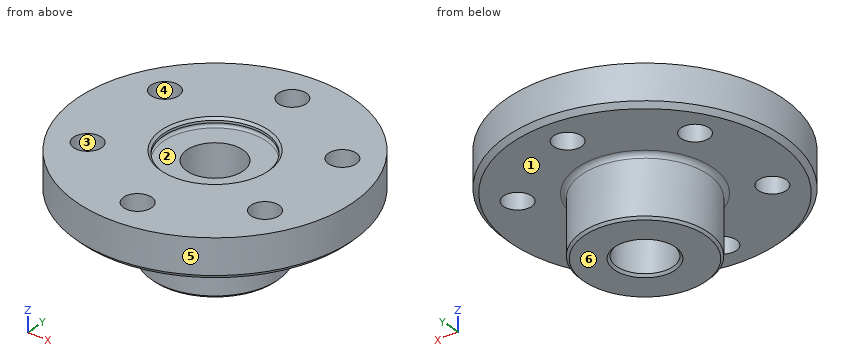
from build123d import *

# Parameters (mm, degrees)
CUT_EXTRUDE1_REACH = 89.396
SKETCH2_R          = 6
CIRPATTERN1_COUNT  = 6
FILLET1_R          = 2
CHAMFER1_SIZE      = 1
CHAMFER2_SIZE      = 2


with BuildPart() as part:
    # Sketch1 → Revolve1 (revolve)
    with BuildSketch(Plane(origin=(0, 0, 0), x_dir=(0, 0, -1), z_dir=(1, 0, 0)), mode=Mode.PRIVATE) as revolve1_sk:
        with BuildLine():
            Line((1.376389422, 12), (1.376389422, 22))
            ThreePointArc((1.376389422, 22), (0.376389422, 23), (-0.623610578, 22))
            Line((-0.623610578, 22), (-2.623610578, 22))
            Line((-2.623610578, 22), (-2.623610578, 59))
            Line((-2.623610578, 59), (14.376389422, 59))
            Line((14.376389422, 59), (14.376389422, 27))
            Line((14.376389422, 27), (40.376389422, 27))
            Line((40.376389422, 27), (40.376389422, 12))
            Line((40.376389422, 12), (1.376389422, 12))
        make_face()
    revolve(revolve1_sk.sketch.rotate(Axis((0, 0, 9.001223373), (0, 0, -1)), 90), axis=Axis((0, 0, 9.001223373), (0, 0, -1)))

    # Sketch2 → Cut-Extrude1 (cut, up to next)
    with BuildSketch(Plane(origin=(0, 0, -14.376389422), x_dir=(-1, 0, 0), z_dir=(0, 0, -1)), mode=Mode.PRIVATE) as cut_extrude1_sk1:
        with Locations((0, 44)):
            Circle(SKETCH2_R)
    cut_extrude1_tool1 = extrude(cut_extrude1_sk1.sketch, amount=-CUT_EXTRUDE1_REACH, mode=Mode.PRIVATE) & part.part
    cut_extrude1 = cut_extrude1_tool1.solids().sort_by_distance((0, 44, -14.376389))[0]
    add(cut_extrude1, mode=Mode.SUBTRACT)

    # CirPattern1: Cut-Extrude1 ×6 about axis
    cirpattern1_axis = Axis((0, 0, 0), (0, 0, 1))
    for i in range(1, CIRPATTERN1_COUNT):
        add(cut_extrude1.rotate(cirpattern1_axis, i * 360 / CIRPATTERN1_COUNT), mode=Mode.SUBTRACT)

    # Fillet1
    fillet1_edges = [part.edges().sort_by_distance(p)[0] for p in [
        (-27, 0, -14.376389422),
    ]]
    fillet(fillet1_edges, radius=FILLET1_R)

    # Chamfer1
    chamfer1_edges = [part.edges().sort_by_distance(p)[0] for p in [
        (-12, 0, -40.376389422),
        (-22, 0, 2.623610578),
        (-27, 0, -40.376389422),
    ]]
    chamfer(chamfer1_edges, length=CHAMFER1_SIZE)

    # Chamfer2
    chamfer2_edges = [part.edges().sort_by_distance(p)[0] for p in [
        (-59, 0, -14.376389422),
    ]]
    chamfer(chamfer2_edges, length=CHAMFER2_SIZE)


solid = part.part
Build history of the part. All positions in model axes, mm. Face numbers are marked on the shaded views. A direction names the side the tool comes from. Round coordinates to 2 decimals unless told otherwise and drop trailing zeros. Loops run counter-clockwise (first coordinate to the right, second up) from the corner with the lowest first, then second, coordinate; pieces in that order, holes last. Notation, with made-up numbers: (29, 67) -> (67, 67) arc R23 cw to (67, 99) -> close; hole circle Ø1 at (-16, -4). An arc over 180 degrees is marked (long way). Use CSV: the item, a comma, the result in double quotes. Start each with the question number.
Q1. Mould opens along Y. For the marked faces 4, 5 and 6 say: +Y half, -Y half, draft (parallel to the pull), parting line (faces both ways), or undercut.
Q2. Saw through at A-A on y = 0. Give the cut face in (x, z).
Q3. Which spindle directions (+Z, -Z, +X, -X, +Y, -Y) get a long thin tool onto all of the face, cutting with end or side? Do the marked faces 1, 2 and 3. Say none if no direction does.
Q4. Saw through at C-C on z = -26.5. Give the cut face in (x, y).
Q5. Flat gauge pins, fed straight in: pin 1 Ø19 at (x, y) = (0, 0) entering from -Z; pin 2 Ø1 at (y, z) = (17.5, -28.5) entering from +X; pin 3 Ø15.5 at (x, y) = (0, 44) entering from -Z; pin 4 Ø6 at (x, z) = (-16.5, -26.5) entering from +Y. Where does each tip first touch, or does it go through?
Q6. Saw through at D-D on z = -3. Give the cut face in (x, y), and give its area (3 significant figures).
Q7. Drill centre lines: L1, parallel to Y at x = 0, z = 1.15; L2, parallel to Y at x = -42, z = 1; L3, parallel to Y at x = 43.5, z = -3.5. Where is each one in solid material? Low to high.
Q8. Saw through at B-B on x = 0. Count the separate pieces of the cut face and the enclosed holes in it, and give its area (3 significant figures).
Solutions:
1,face 4,"undercut"
1,face 5,"parting line"
1,face 6,"draft"
2,outline,"(-59, -12.38) -> (-57, -14.38) -> (-29, -14.38) arc R2 cw to (-27, -16.38) -> (-27, -39.38) -> (-26, -40.38) -> (-13, -40.38) -> (-12, -39.38) -> (-12, -1.38) -> (-22, -1.38) arc R1 cw to (-22, 0.62) -> (-22, 1.62) -> (-23, 2.62) -> (-59, 2.62) -> close; (12, -39.38) -> (13, -40.38) -> (26, -40.38) -> (27, -39.38) -> (27, -16.38) arc R2 cw to (29, -14.38) -> (57, -14.38) -> (59, -12.38) -> (59, 2.62) -> (23, 2.62) -> (22, 1.62) -> (22, 0.62) arc R1 cw to (22, -1.38) -> (12, -1.38) -> close"
3,face 1,"-Z"
3,face 2,"+Z"
3,face 3,"+Z, -Z"
4,outline,"circle Ø54 at (0, 0); hole circle Ø24 at (0, 0)"
5,pin 1,"passes through"
5,pin 2,"stops at x = 20.98"
5,pin 3,"stops at z = -14.38"
5,pin 4,"stops at y = 23.38"
6,outline,"circle Ø118 at (0, 0); hole circle Ø12 at (-38.11, -22); hole circle Ø12 at (-38.11, 22); hole circle Ø24 at (0, 0); hole circle Ø12 at (0, -44); hole circle Ø12 at (0, 44); hole circle Ø12 at (38.11, -22); hole circle Ø12 at (38.11, 22)"
6,area,"9,800 mm^2"
7,L1,"y = -59 to -50, -38 to -22, 22 to 38, 50 to 59"
7,L2,"y = -41.44 to -26.56, -17.44 to 17.44, 26.56 to 41.44"
7,L3,"y = -39.86 to -24.63, -19.37 to 19.37, 24.63 to 39.86"
8,separate pieces,"4"
8,enclosed holes,"0"
8,area,"1,880 mm^2"
